from build123d import *

# Parameters (mm, degrees)
SKETCH1_R           = 4.445
BOSS_EXTRUDE1_DEPTH = 2.1
SKETCH2_R           = 4.7625
BOSS_EXTRUDE2_DEPTH = 2
SKETCH4_R           = 6.35
BOSS_EXTRUDE4_DEPTH = 1.5875
SKETCH5_R           = 3.175
CUT_EXTRUDE1_DEPTH  = 12.375


with BuildPart() as part:
    # Sketch1 → Boss-Extrude1 (new body)
    with BuildSketch(Plane.XY):
        Circle(SKETCH1_R)
    boss_extrude1 = extrude(amount=BOSS_EXTRUDE1_DEPTH)

    # Sketch2 → Boss-Extrude2 (add)
    with BuildSketch(Plane.XY.offset(2.1)):
        Circle(SKETCH2_R)
    boss_extrude2 = extrude(amount=BOSS_EXTRUDE2_DEPTH)

    # Sketch4 → Boss-Extrude4 (add)
    with BuildSketch(Plane.XY.offset(4.1)):
        Circle(SKETCH4_R)
    boss_extrude4 = extrude(amount=BOSS_EXTRUDE4_DEPTH)

    # Mirror1: Boss-Extrude1, Boss-Extrude2, Boss-Extrude4 across plane
    add(boss_extrude1.mirror(Plane.XY))
    add(boss_extrude2.mirror(Plane.XY))
    add(boss_extrude4.mirror(Plane.XY))

    # Sketch5 → Cut-Extrude1 (cut, through all)
    with BuildSketch(Plane.XY.offset(5.6875)):
        Circle(SKETCH5_R)
    extrude(amount=-CUT_EXTRUDE1_DEPTH, mode=Mode.SUBTRACT)


solid = part.part
CAD build for the part. Positions are in the model's coordinates, mm. A direction names the side the tool comes from. Give positions to 0.01 mm unless a question says otherwise; leave off trailing zeros. Loops run counter-clockwise (first coordinate to the right, second up) from the corner with the lowest first, then second, coordinate; pieces in that order, holes last. Notation, with made-up numbers: M 37.5,32 L 51.5,32 A13 ccw 51.5,38 Z; hole C 10.5,32 d5. An arc over 180 degrees is marked long. Write each question's results on one line, items separated by ' | '.
Q1. Which spindle directions (+Z, -Z, +X, -X, +Y, -Y) get a long thin tool onto all of the face, cutting with end or side? Do faces 5 (the face through (-1.38, -6.2, 4.88)), 6 (the face through (1, 5, 4.1)). Say none if no direction does.
Geometry check:
face 5: +Z, -Z | face 6: none
Q2. Band-saw the part on D-D on x = 5. Write the cut outline in (y, z).
Geometry check:
outline: M -3.91,-5.69 L 3.91,-5.69 L 3.91,-4.1 L -3.91,-4.1 Z; M -3.91,4.1 L 3.91,4.1 L 3.91,5.69 L -3.91,5.69 Z
Q3. Flat gauge pins, fed straight in: P1, Ø1.5, axis at y = -4.5, z = 0, coming from the -X side; P2, Ø1.5, axis at x = 0, z = 2, coming from the +Y side. Where does each tip first touch, or does it go through?
Geometry check:
P1: stops at x = -2.39 | P2: stops at y = 4.76
Q4. Mould opens along Z. For faces 1 (the face through (-3.78, -2.9, 3.09)), 2 (the face through (-2, 3, -5.688)), 3 (the face through (-3.78, -2.9, -3.09)), 4 (the face through (-2, 3, 5.688)) say: pulls with the +Z half, pulls with the -Z half, needs draft (parallel to the pull), parting line crosses it, or undercut.
Geometry check:
face 1: undercut | face 2: pulls with the -Z half | face 3: undercut | face 4: pulls with the +Z half
Q5. Band-saw the part on C-C on z = 1. Write the cut outline in (x, y) (3 decimals), and give its area (3 significant figures).
Geometry check:
outline: C 0,0 d8.89; hole C 0,0 d6.35 | area: 30.4 mm²
Q6. Probe probe 1 along Z at (x, y) = (-6, -0.25); probe 2 along Y at (x, z) = (0, 3) (1 decimal); probe 3 along Y at (x, z) = (0, 1.25) (3 decimals). List the from-to ranges inside material, lowest first.
Geometry check:
probe 1: z = -5.69 to -4.1, 4.1 to 5.69 | probe 2: y = -4.8 to -3.2, 3.2 to 4.8 | probe 3: y = -4.445 to -3.175, 3.175 to 4.445
